```python
from build123d import *

# Parameters (mm, degrees)
SKETCH_1_R          = 6
SKETCH_1_R_2        = 2.5
EXTRUDE_1_DEPTH     = 19
SKETCH_2_OUTSIDE_W  = 19.096
SKETCH_2_OUTSIDE_H  = 26.096
SKETCH_2_OUTSIDE_R  = 0.75
CUT_EXTRUDE_1_DEPTH = 9.5
CUT_EXTRUDE_2_DEPTH = 9.5


with BuildPart() as part:
    # 草图1 → 凸台-拉伸1 (new body)
    with BuildSketch(Plane.XY):
        Circle(SKETCH_1_R)
        Circle(SKETCH_1_R_2, mode=Mode.SUBTRACT)
    extrude(amount=EXTRUDE_1_DEPTH)

    # 草图2 outside → 切除-拉伸1 (cut, symmetric)
    with BuildSketch(Plane(origin=(0, 0, 0), x_dir=(1, 0, 0), z_dir=(0, 1, 0))):
        with Locations((0, -9.5)):
            Rectangle(SKETCH_2_OUTSIDE_W, SKETCH_2_OUTSIDE_H)
        with BuildLine():
            Line((-2.75, -2.75), (-2.75, -9))
            ThreePointArc((-2.75, -9), (-3.701902961, -11.298097039), (-6, -12.25))
            Line((-6, -12.25), (-6, -19))
            Line((-6, -19), (6, -19))
            Line((6, -19), (6, -12.25))
            ThreePointArc((6, -12.25), (3.701902961, -11.298097039), (2.75, -9))
            Line((2.75, -9), (2.75, -2.75))
            ThreePointArc((2.75, -2.75), (0, 0), (-2.75, -2.75))
        make_face(mode=Mode.SUBTRACT)
        with Locations((0, -2.75)):
            Circle(SKETCH_2_OUTSIDE_R)
    extrude(amount=CUT_EXTRUDE_1_DEPTH, both=True, mode=Mode.SUBTRACT)

    # 草图3 → 切除-拉伸2 (cut, symmetric)
    with BuildSketch(Plane(origin=(0, 0, 0), x_dir=(0, 0, -1), z_dir=(1, 0, 0))):
        with BuildLine():
            Line((-9.250000001, 3), (0, 3))
            Line((0, 3), (0, -3))
            Line((0, -3), (-9.250000001, -3))
            ThreePointArc((-9.250000001, -3), (-12.250000001, 0), (-9.250000001, 3))
        make_face()
    extrude(amount=CUT_EXTRUDE_2_DEPTH, both=True, mode=Mode.SUBTRACT)


solid = part.part
```
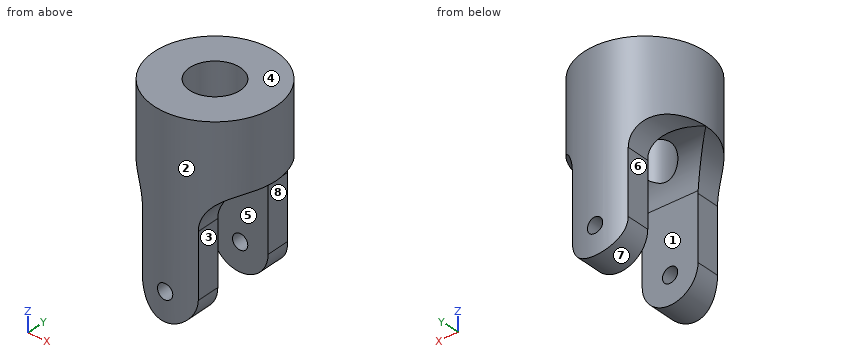
Verification items for the finished model (mm, model axes). Face numbers are marked on the shaded views. A direction names the side the tool comes from. Give positions to 0.01 mm unless a question says otherwise; leave off trailing zeros. Write each loop counter-clockwise with the first axis right and the second up, starting at its lowest first coordinate (ties: lowest second). Pieces come first, ordered by that corner, then holes. Notation, with made-up numbers: M 50,82.25 L 70,82.25 A26 cw 70,104.25 Z; hole C -32,-15.75 d4. An arc over 180 degrees is marked long. One line per question, with ' | ' between items.
1) Mould release check, pull along Y, two halves, no side actions. Record for the marked faces 1, 2 and 3: released by +Y, released by -Y, zero draft, split by the parting line, or undercut.
Result:
face 1: undercut | face 2: split by the parting line | face 3: zero draft
2) Gauge pin test, flat ends, axial feed: pin 1 Ø0.7 at (y, z) = (-4.5, 5) entering from +X; pin 2 Ø1 at (y, z) = (-3.5, 12) entering from -X; pin 3 Ø2.5 at (y, z) = (4.5, 7) entering from -X. Record the tip position at first contact, or that the pin passes through.
Result:
pin 1: stops at x = 2.75 | pin 2: stops at x = -5.18 | pin 3: stops at x = -2.75
3) Set-up check for the marked faces 4, 5, 6, 7 and 8: record each of +Z, -Z, +X, -X, +Y, -Y from which the full face is reachable in a straight line by a thin tool's end or side.
Result:
face 4: +Z, +X, -X, +Y, -Y | face 5: -Z, +X, -X | face 6: -Z, -X, +Y, -Y | face 7: -Z, +Y, -Y | face 8: -Z, +X, +Y, -Y
4) Section check A-A on x = 0. Enter the section's corners in (y, z).
Result:
outline: M -6,0 L -3,0 L -3,2 L -6,2 Z; M -6,3.5 L -3,3.5 L -3,9.25 A3 cw -2.5,10.91 L -2.5,19 L -6,19 Z; M 2.5,10.91 A3 cw 3,9.25 L 3,3.5 L 6,3.5 L 6,19 L 2.5,19 Z; M 3,0 L 6,0 L 6,2 L 3,2 Z
5) Thickness scan on line 1 along X through (y, z) = (-4.15, 2.75); line 2 along Y through (x, z) = (0, 16.5); line 3 along Z through (x, y) = (0, -4.3). Record the ranges inside material, lowest first. Write a range as [from, to].
Result:
line 1: x = [-2.75, -0.75], [0.75, 2.75] | line 2: y = [-6, -2.5], [2.5, 6] | line 3: z = [0, 2], [3.5, 19]
6) Section check B-B on z = 8. Enter the section's corners in (x, y), plus the area to 3 significant figures.
Result:
outline: M -2.75,-5.33 A6 ccw 2.75,-5.33 L 2.75,-3 L -2.75,-3 Z; M -2.75,3 L 2.75,3 L 2.75,5.33 A6 ccw -2.75,5.33 Z | area: 30.6 mm2
7) Section check D-D on x = 2. Enter the section's corners in (y, z), plus the area to 3 significant figures.
Result:
outline: M -5.66,0.86 L -3,0.86 L -3,9.25 A3 cw -1.5,11.85 L -1.5,19 L -5.66,19 Z; M 1.5,11.85 A3 cw 3,9.25 L 3,0.86 L 5.66,0.86 L 5.66,19 L 1.5,19 Z | area: 120 mm2
8) Section check C-C on y = -1.5. Enter the section's corners in (x, z).
Result:
outline: M -5.81,12.24 A3.25 cw -4.43,11.85 L -2,11.85 L -2,19 L -5.81,19 Z; M 2,11.85 L 4.43,11.85 A3.25 cw 5.81,12.24 L 5.81,19 L 2,19 Z
